Verification items for the finished model (mm, model axes). A direction names the side the tool comes from. Give positions to 0.01 mm unless a question says otherwise; leave off trailing zeros. Order: outer loops, then holes, each group sorted by start corner. A loop starts at its lowest first (then second) coordinate and runs counter-clockwise, first axis right, second up. Notation, with made-up numbers: (9.5, -16) - (25.5, -16) arc R30 cw to (25.5, 9) - close; hole circle Ø2 at (36, -26). An arc over 180 degrees is marked (long way). Answer as a JSON object with one key per item and string values.
```python
from build123d import *

# Parameters (mm, degrees)
SKETCH1_R           = 1.3
SKETCH1_W           = 10
SKETCH1_H           = 3
SKETCH1_W_2         = 3
SKETCH1_H_2         = 4.6
BOSS_EXTRUDE1_DEPTH = 3


with BuildPart() as part:
    # Sketch1 → Boss-Extrude1 (new body)
    with BuildSketch(Plane(origin=(0, 0, 0), x_dir=(1, 0, 0), z_dir=(0, 1, 0))):
        with BuildLine():
            Line((0, -20), (0, 103))
            ThreePointArc((0, 103), (1.464466094, 106.535533906), (5, 108))
            Line((5, 108), (55, 108))
            ThreePointArc((55, 108), (58.535533906, 106.535533906), (60, 103))
            Line((60, 103), (60, -20))
            ThreePointArc((60, -20), (58.535533906, -23.535533906), (55, -25))
            Line((55, -25), (5, -25))
            ThreePointArc((5, -25), (1.464466094, -23.535533906), (0, -20))
        make_face()
        with Locations((56.07, 48.068886064)):
            Circle(SKETCH1_R, mode=Mode.SUBTRACT)
        with Locations((4, 15.048886064)):
            Circle(SKETCH1_R, mode=Mode.SUBTRACT)
        with Locations((56.07, 20.128886064)):
            Circle(SKETCH1_R, mode=Mode.SUBTRACT)
        with Locations((5.27, 63.308886064)):
            Circle(SKETCH1_R, mode=Mode.SUBTRACT)
        with Locations((16, 102.5)):
            Rectangle(SKETCH1_W, SKETCH1_H, mode=Mode.SUBTRACT)
        with Locations((44, 102.5)):
            Rectangle(SKETCH1_W, SKETCH1_H, mode=Mode.SUBTRACT)
        with Locations((5.8, 97.3)):
            Rectangle(SKETCH1_W_2, SKETCH1_H_2, mode=Mode.SUBTRACT)
        with Locations((5.8, 70.2)):
            Rectangle(SKETCH1_W_2, SKETCH1_H_2, mode=Mode.SUBTRACT)
        with Locations((54.2, 70.2)):
            Rectangle(SKETCH1_W_2, SKETCH1_H_2, mode=Mode.SUBTRACT)
        with Locations((54.2, 97.3)):
            Rectangle(SKETCH1_W_2, SKETCH1_H_2, mode=Mode.SUBTRACT)
        with Locations((5.8, 8.8)):
            Rectangle(SKETCH1_W_2, SKETCH1_H_2, mode=Mode.SUBTRACT)
        with Locations((5.8, -18.3)):
            Rectangle(SKETCH1_W_2, SKETCH1_H_2, mode=Mode.SUBTRACT)
        with Locations((54.2, 8.8)):
            Rectangle(SKETCH1_W_2, SKETCH1_H_2, mode=Mode.SUBTRACT)
        with Locations((54.2, -18.3)):
            Rectangle(SKETCH1_W_2, SKETCH1_H_2, mode=Mode.SUBTRACT)
    extrude(amount=BOSS_EXTRUDE1_DEPTH)


solid = part.part
```
(1) Section check B-B (y = 2.3). Count the separate pieces of the cut face and the enclosed holes in it, then the cut area to 3 significant figures.
Computed values:
{"separate pieces": "1", "enclosed holes": "14", "area": "7,770 mm²"}
(2) Access from +Z, -Z, +X, -X, +Y, -Y to the whole of each face (thin tool, end or side, straight path). Record for faces 4 (the flat face through (16, 1, -101)), 5 (the flat face through (30, 0, -42)).
Computed values:
{"face 4": "+Y, -Y", "face 5": "+Z, -Z, +X, -X, -Y"}
(3) Section check A-A (x = 41). Record the cut outline in (y, z), then the cut area to 3 significant figures.
Computed values:
{"outline": "(0, -108) - (3, -108) - (3, -104) - (0, -104) - close; (0, -101) - (3, -101) - (3, 25) - (0, 25) - close", "area": "390 mm²"}
(4) Material ranges on line 1 along X through (y, z) = (1.25, -68.5); line 2 along Z through (x, y) = (45, 0.75); line 3 along Z through (x, y) = (56.07, 0.6), recorded low to high. Write a range as [from, to].
Computed values:
{"line 1": "x = [0, 4.3], [7.3, 52.7], [55.7, 60]", "line 2": "z = [-108, -104], [-101, 25]", "line 3": "z = [-107.88, -49.37], [-46.77, -21.43], [-18.83, 24.88]"}
(5) Release check for a two-part mould opening along X. For faces 1 (the cylindrical face through (58, 1, -107)), 2 (the flat face through (30, 1, 25)), 3 (the flat face through (54, 1, -72.5)) record: pulls with the +X half, pulls with the -X half, needs draft (parallel to the pull), parting line crosses it, or undercut.
Computed values:
{"face 1": "pulls with the +X half", "face 2": "needs draft", "face 3": "undercut"}
(6) Gauge pin test, flat end, axial feed: pin 1 Ø2 at (x, z) = (4, -15.05) entering from -Y. Record the tip position at first contact, or that the pin passes through.
Computed values:
{"pin 1": "passes through"}
